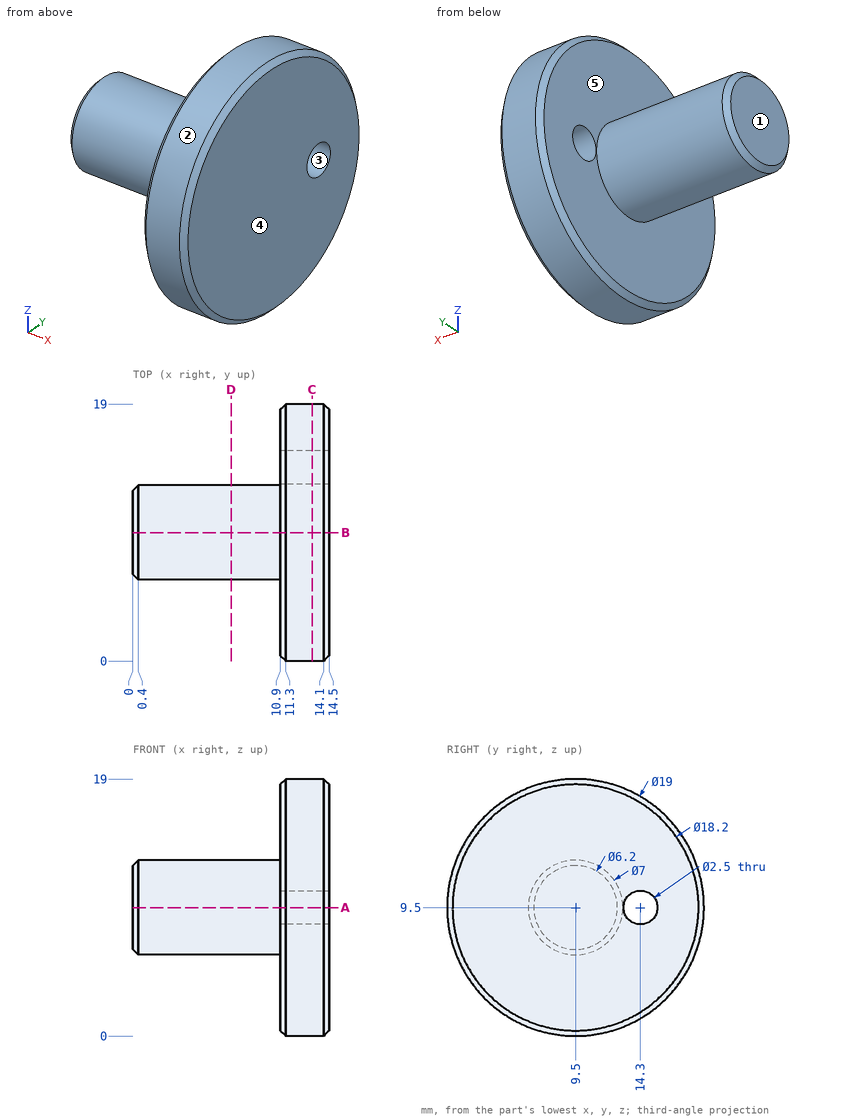
Can you work these out from the drawing? Everything is in mm from the part's minimum corner. A direction names the side the tool comes from. Round coordinates to 2 decimals unless told otherwise and drop trailing zeros. Order: outer loops, then holes, each group sorted by start corner. A loop starts at its lowest first (then second) coordinate and runs counter-clockwise, first axis right, second up.
(1) If I drill on L1, parallel to Y at x = 11.7, z = 9.5; L2, parallel to X at y = 10.5, z = 18.25; L3, parallel to Z at x = 12.5, y = 6, over which ranges is the centre line in solid material (lowest first)?
Results are:
L1: y = 0 to 13.05, 15.55 to 19
L2: x = 10.9 to 14.5
L3: z = 0.67 to 18.33
(2) If we section it at D-D (x = 7.25): Please give me the cut outline in (y, z).
Results are:
outline: circle Ø7 at (9.5, 9.5)
(3) On a 3-axis mill with a long thin cutter (end or side, diameter ignored), from which of +Z, -Z, +X, -X, +Y, -Y can I reach the whole of each face in a straight line? I mean the marked faces 4 and 5. Say none if no direction works.
Results are:
face 4: +Z, -Z, +X, +Y, -Y
face 5: -X
(4) We'd pull the mould along Z, two halves only. Please class the marked faces 1, 2 and 3: +Z half, -Z half, draft (parallel to the pull), parting line (faces both ways), or undercut.
Results are:
face 1: draft
face 2: parting line
face 3: undercut
(5) I'm going to push flat-ended pins straight in: pin 1 (4 mm diameter, centred on x = 10, z = 12, fed in from -Y); pin 2 (3 mm diameter, centred on y = 14.3, z = 9.5, fed in from -X); pin 3 (2 mm diameter, centred on y = 2.5, z = 7, fed in from -X). Where does each tip first touch, or does it pass through?
Results are:
pin 1: stops at y = 0.05
pin 2: stops at x = 0.2
pin 3: stops at x = 10.9
(6) If we section it at C-C (x = 13.25): Please give me the cut outline in (y, z).
Results are:
outline: circle Ø19 at (9.5, 9.5); hole circle Ø2.5 at (14.3, 9.5)
(7) If we section it at B-B (y = 9.5): Please give me the cut outline in (x, z), plus the area to 3 significant figures.
Results are:
outline: (0, 6.4) - (0.4, 6) - (10.9, 6) - (10.9, 0.4) - (11.3, 0) - (14.1, 0) - (14.5, 0.4) - (14.5, 18.6) - (14.1, 19) - (11.3, 19) - (10.9, 18.6) - (10.9, 13) - (0.4, 13) - (0, 12.6) - close
area: 144 mm2
(8) If we section it at A-A (z = 9.5): Please give me the cut outline in (x, y).
Results are:
outline: (0, 6.4) - (0.4, 6) - (10.9, 6) - (10.9, 0.4) - (11.3, 0) - (14.1, 0) - (14.5, 0.4) - (14.5, 13.05) - (10.9, 13.05) - (10.9, 13) - (0.4, 13) - (0, 12.6) - close; (10.9, 15.55) - (14.5, 15.55) - (14.5, 18.6) - (14.1, 19) - (11.3, 19) - (10.9, 18.6) - close
